from build123d import *

# Parameters (mm, degrees)
BOSS_EXTRUDE1_DEPTH = 6.35
FILLET1_R           = 25.4


with BuildPart() as part:
    # Sketch1 → Boss-Extrude1 (new body)
    with BuildSketch(Plane.XY):
        with BuildLine():
            Line((203.2, -228.6), (203.2, -261.62))
            ThreePointArc((203.2, -261.62), (210.639487758, -279.580512242), (228.6, -287.02))
            Line((228.6, -287.02), (393.671225938, -287.02))
            ThreePointArc((393.671225938, -287.02), (519.394811633, -234.943585695), (571.471225938, -109.22))
            Line((571.471225938, -109.22), (571.471225938, 55.88))
            Line((571.471225938, 55.88), (537.728452035, 55.88))
            ThreePointArc((537.728452035, 55.88), (511.766359552, 48.744742687), (493.097424953, 29.343376138))
            ThreePointArc((493.097424953, 29.343376138), (370.666792044, -124.935933237), (203.2, -228.6))
        make_face()
    extrude(amount=BOSS_EXTRUDE1_DEPTH)

    # Fillet1
    fillet1_edges = [part.edges().sort_by_distance(p)[0] for p in [
        (203.2, -228.6, 3.175),
    ]]
    fillet(fillet1_edges, radius=FILLET1_R)


solid = part.part
Can you work these out from the model? Positions are in its coordinate system, mm. Round coordinates to 2 decimals unless told otherwise and drop trailing zeros. Write each loop counter-clockwise with the first axis right and the second up, starting at its lowest first coordinate (ties: lowest second). Pieces come first, ordered by that corner, then holes. Notation, with made-up numbers: (77.25, 3.5) - (95.25, 3.5) arc R18 cw to (95.25, 14.5) - close; hole circle Ø7 at (42, 2.25). An arc over 180 degrees is marked (long way). Write each question's results on one line, items separated by ' | '. Start each with the question number.
1) Suppose I cut it at A-A (z = 5). List the corners of the cut face in (x, y) for me.
2) For pin 1 Ø3 at (y, z) = (-5.5, 1) entering from -X; pin 2 Ø1 at (y, z) = (-161.5, 3.5) entering from +X, each with a flat end and sliding along its axis, tell me the tip position at first contact or that it passes through.
3) Please list where these lines run through material, in increasing order: line 1 (Y direction, x = 337, z = 3.5); line 2 (Y direction, x = 331, z = 4.5); line 3 (X direction, y = -162.5, z = 0.75).
4) Suppose I cut it at B-B (x = 438). List the corners of the cut face in (y, z) for me, and give its area (3 significant figures).
5) Suppose I cut it at C-C (y = -135.5). List the corners of the cut face in (x, z) for me.
Here are the results:
1) outline: (203.2, -261.62) arc R25.4 ccw to (228.6, -287.02) - (393.67, -287.02) arc R177.8 ccw to (571.47, -109.22) - (571.47, 55.88) - (537.73, 55.88) arc R50.8 ccw to (493.1, 29.34) arc R572.56 cw to (218.47, -222.22) arc R25.4 ccw to (203.2, -245.51) - close
2) pin 1: stops at x = 471.57 | pin 2: stops at x = 563.76
3) line 1: y = -287.02 to -152.67 | line 2: y = -287.02 to -157.18 | line 3: x = 323.7 to 563.3
4) outline: (-281.41, 0) - (-53.81, 0) - (-53.81, 6.35) - (-281.41, 6.35) - close | area: 1,450 mm2
5) outline: (358.45, 0) - (569.52, 0) - (569.52, 6.35) - (358.45, 6.35) - close
